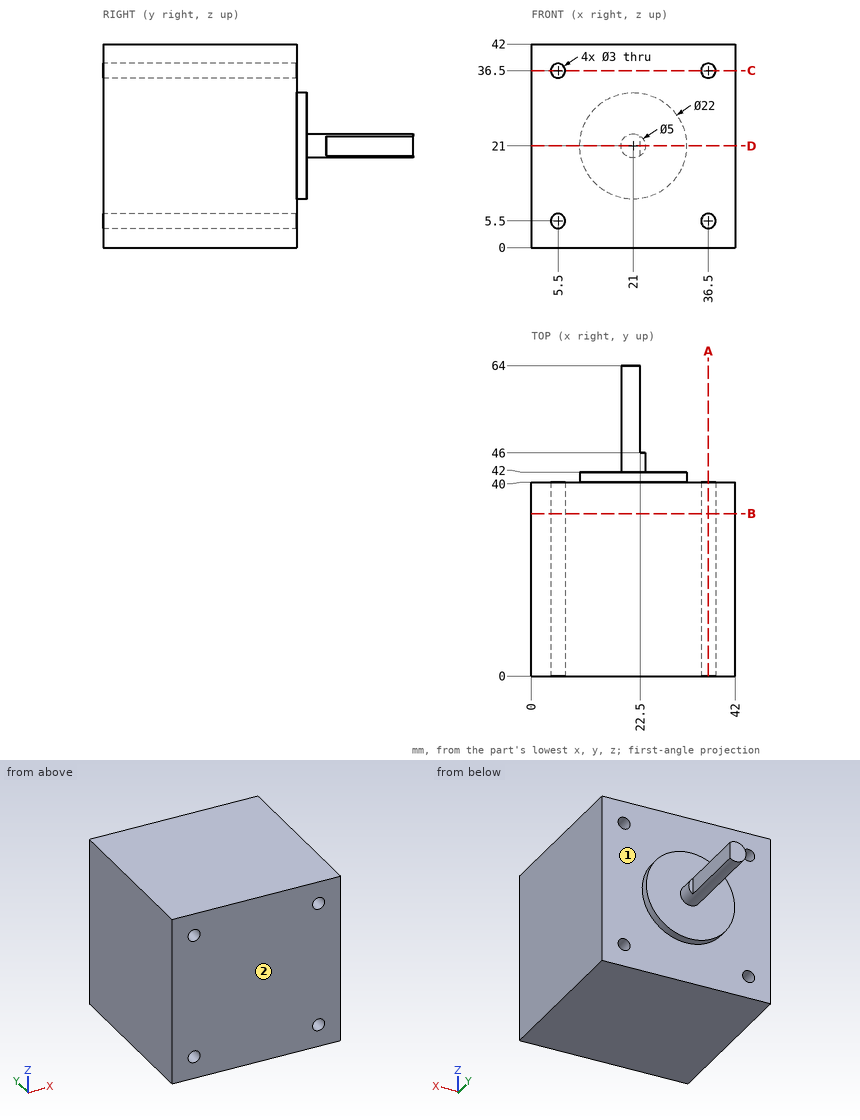
Design review of the part shown in the three views and the two pictorial views. Dimensions are in mm from the part's minimum x, y and z. A direction names the side the tool comes from. Round coordinates to 2 decimals unless told otherwise and drop trailing zeros. Loops run counter-clockwise (first coordinate to the right, second up) from the corner with the lowest first, then second, coordinate; pieces in that order, holes last.
(1) Clearance check with flat-ended pins moving along their axes: P1, Ø3.5, axis at x = 36.5, z = 5.5, coming from the +Y side; P2, Ø3, axis at y = 59, z = 20.5, coming from the +X side; P3, Ø4, axis at x = 18.5, y = 51, coming from the +Z side; P4, Ø2, axis at y = 41.5, z = 6, coming from the +X side (1 decimal). State where each tip first meets the part, or that it passes through.
Returned:
P1: stops at y = 40
P2: stops at x = 22.5
P3: stops at z = 23.45
P4: passes through
(2) We need section B-B (y = 33.5). Give the boundary of the cut face in (x, z).
Returned:
outline: (0, 0) - (42, 0) - (42, 42) - (0, 42) - close; hole circle Ø3 at (5.5, 5.5); hole circle Ø3 at (5.5, 36.5); hole circle Ø3 at (36.5, 5.5); hole circle Ø3 at (36.5, 36.5)
(3) We need section C-C (z = 36.5). Give the boundary of the cut face in (x, y).
Returned:
outline: (0, 0) - (4, 0) - (4, 40) - (0, 40) - close; (7, 0) - (35, 0) - (35, 40) - (7, 40) - close; (38, 0) - (42, 0) - (42, 40) - (38, 40) - close
(4) Wall thickness on line 1 along X through (y, z) = (30, 5.5); line 2 along Z through (x, y) = (5, 15): over which ranges is each line inside the solid? List them lowest first.
Returned:
line 1: x = 0 to 4, 7 to 35, 38 to 42
line 2: z = 0 to 4.09, 6.91 to 35.09, 37.91 to 42
(5) We need section A-A (x = 36.5). Give the boundary of the cut face in (y, z).
Returned:
outline: (0, 0) - (40, 0) - (40, 4) - (0, 4) - close; (0, 7) - (40, 7) - (40, 35) - (0, 35) - close; (0, 38) - (40, 38) - (40, 42) - (0, 42) - close
(6) We need section D-D (z = 21). Give the boundary of the cut face in (x, y), plus the area to 3 significant figures.
Returned:
outline: (0, 0) - (42, 0) - (42, 40) - (32, 40) - (32, 42) - (23.5, 42) - (23.5, 46) - (22.5, 46) - (22.5, 64) - (18.5, 64) - (18.5, 42) - (10, 42) - (10, 40) - (0, 40) - close
area: 1,820 mm2
(7) Tool access review of the marked faces 1 and 2: name each direction out of +Z, -Z, +X, -X, +Y, -Y from which nothing blocks a thin tool from reaching the whole face with its end or side.
Returned:
face 1: +Y
face 2: +Z, -Z, +X, -X, -Y
